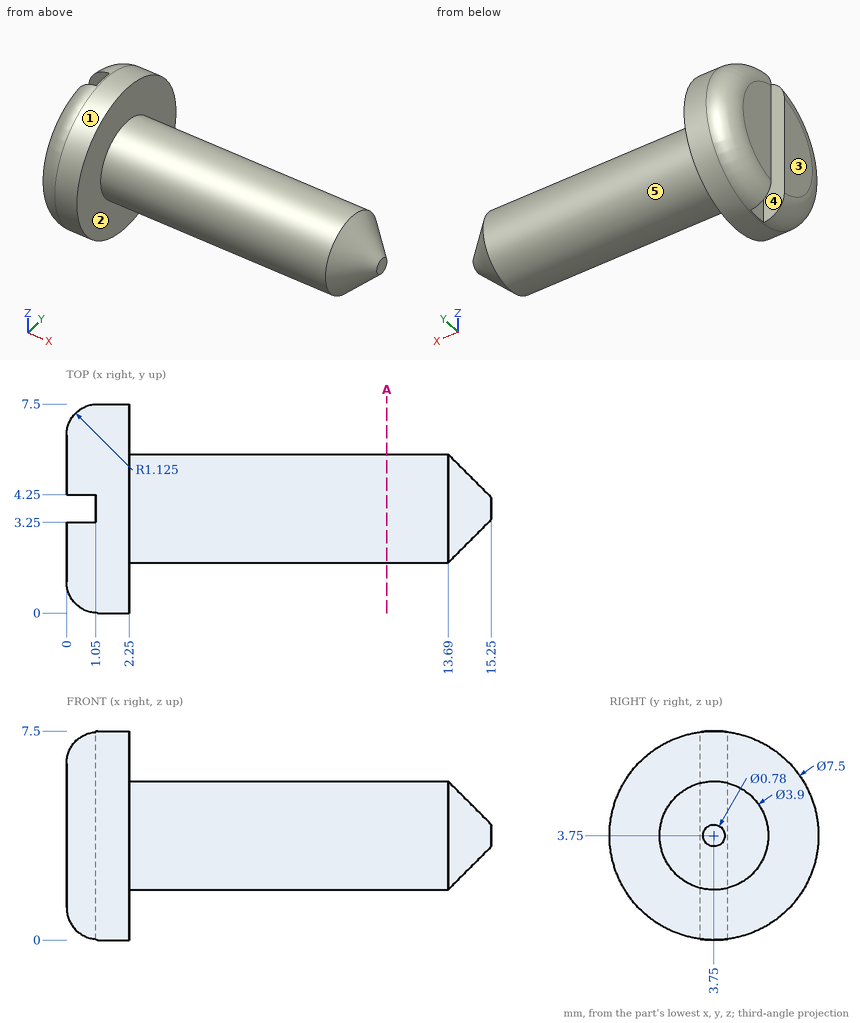
Geometry check sheet. Reference: drawing and pictorial views, mm from the part's lowest x, y, z. A direction names the side the tool comes from. Give positions to 0.01 mm unless a question says otherwise; leave off trailing zeros. Order: outer loops, then holes, each group sorted by start corner. A loop starts at its lowest first (then second) coordinate and runs counter-clockwise, first axis right, second up. Notation, with made-up numbers: M 27,17.25 L 44,17.25 A20 ccw 44,50.25 Z; hole C 87.25,66 d1. An arc over 180 degrees is marked long. Answer as a JSON object with one key per item and string values. Group by question number.
1) Cross-section at A-A (x = 11.5). Enter the section's corners in (y, z), then the cut area to 3 significant figures.
2) Mould release check, pull along Y, two halves, no side actions. Record for the marked faces 3, 4 and 5: released by +Y, released by -Y, zero draft, split by the parting line, or undercut.
3) Access from +Z, -Z, +X, -X, +Y, -Y to the whole of each face (thin tool, end or side, straight path). Record for the marked faces 1 and 2.
4) Depth check by flat-ended pin: pin 1 Ø2 at (y, z) = (5.5, 4) entering from +X; pin 2 Ø1.5 at (x, y) = (5.5, 6) entering from +Z; pin 3 Ø1.5 at (x, z) = (8.5, 6) entering from +Y. Enter the tip coordinate at first touch or a pass-through.
5) Scan lines: line 1 along Y through (x, z) = (1, 0.5); line 2 along Y through (x, z) = (0.75, 6.75); line 3 along X through (y, z) = (4.75, 5.5). Record each from-to range of solid material in increasing order. Write a range as [from, to].
Result sheet:
{
 "1": {"outline": "C 3.75,3.75 d3.9", "area": "11.9 mm2"},
 "2": {"face 3": "zero draft", "face 4": "undercut", "face 5": "split by the parting line"},
 "3": {"face 1": "+X, -X", "face 2": "+X"},
 "4": {"pin 1": "stops at x = 14.87", "pin 2": "stops at z = 5", "pin 3": "stops at y = 5"},
 "5": {"line 1": "y = [1.89, 3.25], [4.25, 5.61]", "line 2": "y = [1.61, 3.25], [4.25, 5.89]", "line 3": "x = [0, 2.25]"}
}
